CAD build for the part. Positions are in the model's coordinates, mm. A direction names the side the tool comes from. Coordinates: 2 decimals unless noted, no trailing zeros. Loops run counter-clockwise (first coordinate to the right, second up) from the corner with the lowest first, then second, coordinate; pieces in that order, holes last. Notation, with made-up numbers: (22, -14) - (58, -14) arc R13 cw to (58, -3) - close; hole circle Ø9 at (46.25, 24.25). An arc over 180 degrees is marked (long way). Put each result on its own line as item: value.
```python
from build123d import *

# Parameters (mm, degrees)
F1_DEPTH  = 3.175
F3_DEPTH  = 7.62
F5_DEPTH  = 7.62
F7_DEPTH  = 40.64
F8_R      = 1.5875
F9_DEPTH  = 25.4
F10_DEPTH = 25.4


with BuildPart() as f1:
    # F0 (on Top) → F1 (new body)
    with BuildSketch(Plane.XY):
        with BuildLine():
            Line((25.9830465623, -3.06), (32.3330465623, 3.29))
            ThreePointArc((32.3330465623, 3.29), (0, 32.5), (-32.3330465623, 3.29))
            Line((-32.3330465623, 3.29), (-25.9830465623, -3.06))
            Line((-25.9830465623, -3.06), (0, -3.06))
            Line((0, -3.06), (25.9830465623, -3.06))
        make_face()
    extrude(amount=F1_DEPTH)

    # F2 (on face) → F3 (join)
    with BuildSketch(Plane.XY.offset(3.175)):
        with BuildLine():
            Line((15.24, 2.02), (15.24, 28.7052678092))
            ThreePointArc((15.24, 28.7052678092), (0, 32.5), (-15.24, 28.7052678092))
            Line((-15.24, 28.7052678092), (-15.24, 2.02))
            Line((-15.24, 2.02), (15.24, 2.02))
        make_face()
    extrude(amount=F3_DEPTH)

    # F4 (on face) → F5 (cut)
    with BuildSketch(Plane.XY.offset(10.795)):
        with BuildLine():
            ThreePointArc((7.62, 31.594075394), (5.0959805235, 32.0979903188), (2.54, 32.4005925872))
            Line((2.54, 32.4005925872), (2.54, 5.195))
            Line((2.54, 5.195), (7.62, 5.195))
            Line((7.62, 5.195), (7.62, 31.594075394))
        make_face()
        with BuildLine():
            Line((-2.54, 5.195), (-2.54, 32.4005925872))
            ThreePointArc((-2.54, 32.4005925872), (-5.0959805235, 32.0979903188), (-7.62, 31.594075394))
            Line((-7.62, 31.594075394), (-7.62, 5.195))
            Line((-7.62, 5.195), (-2.54, 5.195))
        make_face()
    extrude(amount=-F5_DEPTH, mode=Mode.SUBTRACT)

    # F6 (on face) → F7 (join)
    with BuildSketch(Plane.XY.offset(10.795)):
        with BuildLine():
            Line((-10.16, 2.02), (-10.16, 30.8710932751))
            ThreePointArc((-10.16, 30.8710932751), (-12.7460856731, 29.896275688), (-15.24, 28.7052678092))
            Line((-15.24, 28.7052678092), (-15.24, 2.02))
            Line((-15.24, 2.02), (-10.16, 2.02))
        make_face()
        with BuildLine():
            Line((10.16, 30.8710932751), (10.16, 2.02))
            Line((10.16, 2.02), (15.24, 2.02))
            Line((15.24, 2.02), (15.24, 28.7052678092))
            ThreePointArc((15.24, 28.7052678092), (12.7460856731, 29.896275688), (10.16, 30.8710932751))
        make_face()
    extrude(amount=F7_DEPTH)

    # F8 (on face) → F9 (cut)
    with BuildSketch(Plane(origin=(0, 5.195, 0), x_dir=(-1, 0, 0), z_dir=(0, 1, 0))):
        with Locations((-5.08, 6.985)):
            Circle(F8_R)
        with Locations((5.08, 6.985)):
            Circle(F8_R)
    extrude(amount=-F9_DEPTH, mode=Mode.SUBTRACT)

    # F8 (on face) → F10 (cut)
    with BuildSketch(Plane(origin=(0, 5.195, 0), x_dir=(-1, 0, 0), z_dir=(0, 1, 0))):
        with Locations((5.08, 6.985)):
            Circle(F8_R)
    extrude(amount=-F10_DEPTH, mode=Mode.SUBTRACT)


solid = f1.part
```
Q1. Slice it at B-B, the plane y = 30. Give the cut face in (x, z) (3 decimals), then the cut area to 3 significant figures.
Determined:
outline: (-12.5, 0) - (12.5, 0) - (12.5, 51.435) - (10.16, 51.435) - (10.16, 10.795) - (7.62, 10.795) - (7.62, 3.175) - (2.54, 3.175) - (2.54, 10.795) - (-2.54, 10.795) - (-2.54, 3.175) - (-7.62, 3.175) - (-7.62, 10.795) - (-10.16, 10.795) - (-10.16, 51.435) - (-12.5, 51.435) - close
area: 383 mm2
Q2. Slice it at A-A, the plane z = 12. Give the cut face in (x, y), then the cut area to 3 significant figures.
Determined:
outline: (-15.24, 2.02) - (-10.16, 2.02) - (-10.16, 30.87) arc R32.5 ccw to (-15.24, 28.71) - close; (10.16, 2.02) - (15.24, 2.02) - (15.24, 28.71) arc R32.5 ccw to (10.16, 30.87) - close
area: 283 mm2
Q3. Slice it at D-D, the plane x = -11.5. Give the cut face in (y, z) (3 decimals), then the cut area to 3 significant figures.
Determined:
outline: (-3.06, 0) - (30.397, 0) - (30.397, 51.435) - (2.02, 51.435) - (2.02, 3.175) - (-3.06, 3.175) - close
area: 1,480 mm2
Q4. Pin check, flat tips, straight feed: pin 1 Ø10 at (x, y) = (-4, 10.5) entering from +Z (3 decimals); pin 2 Ø2.5 at (y, z) = (21.5, 6) entering from +X; pin 3 Ø1.5 at (x, y) = (5, 15.5) entering from +Z (3 decimals). Stop position of each tip, or through.
Determined:
pin 1: z = 10.795
pin 2: x = 15.24
pin 3: z = 3.175
Q5. Wall check: L1, parallel to X at y = 19.5, z = 11; L2, parallel to Z at x = 5, y = 3 (3 decimals); L3, parallel to Z at x = -7, y = 18 (3 decimals). Give the ranges that are in metal, low to high. Write a range as from..to.
Determined:
L1: -15.24..-10.16, 10.16..15.24
L2: 0..5.4, 8.57..10.795
L3: 0..3.175
Q6. Tool access for faces 1 (the flat face through (-7, 5.195, 7)), 2 (the flat face through (2, 1, 3.175)), 3 (the flat face through (-10.4, 2.02, 21.6)): list every direction of +Z, -Z, +X, -X, +Y, -Y with a clear straight run to the whole face (end or side of a thin tool).
Determined:
face 1: +Z, +Y
face 2: +Z, -Y
face 3: +Z, +X, -X, -Y
Q7. Slice it at C-C, the plane x = 5.08. Give the cut face in (y, z) (1 decimal), then the cut area to 3 significant figures.
Determined:
outline: (-3.1, 0) - (32.1, 0) - (32.1, 3.2) - (5.2, 3.2) - (5.2, 5.4) - (2, 5.4) - (2, 3.2) - (-3.1, 3.2) - close; (2, 8.6) - (5.2, 8.6) - (5.2, 10.8) - (2, 10.8) - close
area: 126 mm2
Q8. Mould opens along X. For faces 4 (the flat face through (5, 19, 3.175)), 5 (the flat face through (-13, 17, 51.435)), 6 (the flat face through (15.24, 15, 27)), 7 (the flat face through (7, 5.195, 7)) say: +X half, -X half, draft (parallel to the pull), parting line (faces both ways), or undercut.
Determined:
face 4: undercut
face 5: draft
face 6: +X half
face 7: undercut
